Source: three-view drawing plus pictorial views. Frame: mm from the lowest corner of the part. A direction names the side the tool comes from. Round coordinates to 2 decimals unless told otherwise and drop trailing zeros. Loops run counter-clockwise (first coordinate to the right, second up) from the corner with the lowest first, then second, coordinate; pieces in that order, holes last. Notation, with made-up numbers: (-10, 3.25) -> (37, 3.25) arc R14 ccw to (37, 28.25) -> close; hole circle Ø7 at (-39, 50). An arc over 180 degrees is marked (long way). Answer in a Markdown table with one row per item. Add a question column.
Q1. Section D-D, the plane x = 20. Output: boundary loops of the cut face in (y, z), and give its area (3 significant figures).
Q2. Section B-B, the plane y = 6.75. Output: boundary loops of the cut face in (x, z).
Q3. Mould query, pull axis X, two halves, no side actions, for the marked faces 1, 2 and 3. Classes: pulls with the +X half, pulls with the -X half, needs draft (parallel to the pull), parting line crosses it, or undercut.
Q4. Pin query (flat end, axial travel): pin 1 (1.2 mm diameter, centred on x = 3, y = 2.5, fed in from -Z); pin 2 (1 mm diameter, centred on x = 5, y = 4.5, fed in from -Z) (1 decimal); pin 3 (1.5 mm diameter, centred on y = 8.5, z = 12.5, fed in from +X). Return the tip coordinate at first contact, or that it passes through.
Q5. Ray query, L1, parallel to Z at x = 3.5, y = 2.5; L2, parallel to X at y = 1.75, z = 5; L3, parallel to X at y = 6.5, z = 8. Return the intervals inside material, ascending. Write a range as from..to.
Q6. Section C-C, the plane z = 8. Output: boundary loops of the cut face in (x, y).
Q7. Section A-A, the plane z = 4.5. Output: boundary loops of the cut face in (x, y), and give its area (3 significant figures).
Q8. Reachability of the marked faces 4, 5 and 6 from +Z, -Z, +X, -X, +Y, -Y: full face, straight path, thin tool, end or side. Return the list, or none.
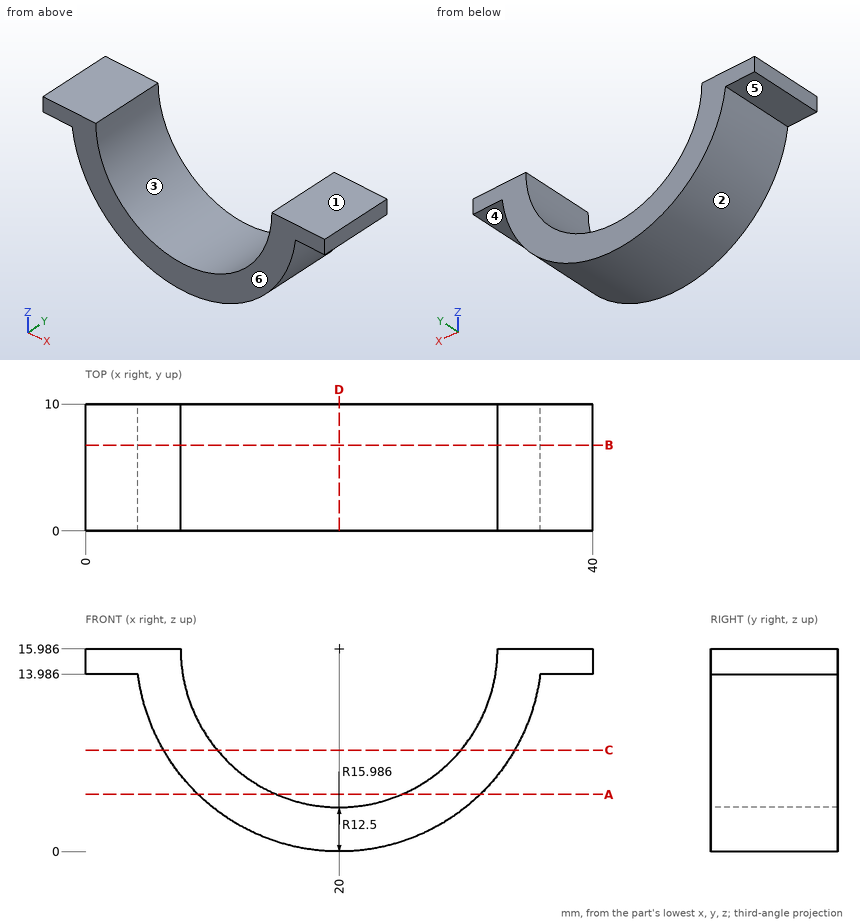
Answer block:
| question | item | result |
|---|---|---|
| 1 | outline | (0, 0) -> (10, 0) -> (10, 3.49) -> (0, 3.49) -> close |
| 1 | area | 34.9 mm^2 |
| 2 | outline | (0, 13.99) -> (4.14, 13.99) arc R15.99 ccw to (35.86, 13.99) -> (40, 13.99) -> (40, 15.99) -> (32.5, 15.99) arc R12.5 cw to (7.5, 15.99) -> (0, 15.99) -> close |
| 3 | face 1 | needs draft |
| 3 | face 2 | parting line crosses it |
| 3 | face 3 | undercut |
| 4 | pin 1 | z = 13.99 |
| 4 | pin 2 | z = 9.3 |
| 4 | pin 3 | x = 35.75 |
| 5 | L1 | 13.99..15.99 |
| 5 | L2 | 8.39..14.04, 25.96..31.61 |
| 5 | L3 | 6.15..10.38, 29.62..33.85 |
| 6 | outline | (6.15, 0) -> (10.38, 0) -> (10.38, 10) -> (6.15, 10) -> close; (29.62, 0) -> (33.85, 0) -> (33.85, 10) -> (29.62, 10) -> close |
| 7 | outline | (8.88, 0) -> (15.07, 0) -> (15.07, 10) -> (8.88, 10) -> close; (24.93, 0) -> (31.12, 0) -> (31.12, 10) -> (24.93, 10) -> close |
| 7 | area | 124 mm^2 |
| 8 | face 4 | -Z, +X, +Y, -Y |
| 8 | face 5 | -Z, -X, +Y, -Y |
| 8 | face 6 | +Z, -Z, +X, -X, -Y |
